Source: CAD feature listing. Evaluate the final solid. Frame: model axes, mm. Give positions to 0.01 mm unless a question says otherwise; leave off trailing zeros. Order: outer loops, then holes, each group sorted by start corner. A loop starts at its lowest first (then second) coordinate and runs counter-clockwise, first axis right, second up. Notation, with made-up numbers: (40, 49) -> (95, 49) arc R16 cw to (95, 76) -> close; hole circle Ø10 at (-37.75, -40). An arc over 180 degrees is marked (long way). Use CSV: the item, a comma, the result in double quotes.
```python
from build123d import *

# Parameters (mm, degrees)
F0_W     = 381
F0_H     = 381
F1_DEPTH = 2.54
F2_R     = 19.05
F3_DEPTH = 2.541


with BuildPart() as f1:
    # F0 (on Front) → F1 (new body)
    with BuildSketch(Plane.XZ):
        with Locations((1.796125, 1.474147)):
            Rectangle(F0_W, F0_H)
    extrude(amount=F1_DEPTH)

    # F2 (on face) → F3 (cut, through all)
    with BuildSketch(Plane.XZ.offset(2.54)):
        Circle(F2_R)
        with Locations((-84.602214, -27.307058)):
            Circle(F2_R)
    extrude(amount=-F3_DEPTH, mode=Mode.SUBTRACT)


solid = f1.part
```
1. Pin query (flat end, axial travel): P1, Ø8, axis at x = -91.5, z = 92.5, coming from the +Y side. Return the tip coordinate at first contact, or that it passes through.
Answer below:
P1,"stops at y = 0"
2. Section query B-B on x = 0. Return loops of the section in (y, z), plus the area to 3 significant figures.
Answer below:
outline,"(-2.54, -189.03) -> (0, -189.03) -> (0, -19.05) -> (-2.54, -19.05) -> close; (-2.54, 19.05) -> (0, 19.05) -> (0, 191.97) -> (-2.54, 191.97) -> close"
area,"871 mm²"
3. Section query A-A on z = 0. Return loops of the section in (x, y).
Answer below:
outline,"(-188.7, -2.54) -> (-19.05, -2.54) -> (-19.05, 0) -> (-188.7, 0) -> close; (19.05, -2.54) -> (192.3, -2.54) -> (192.3, 0) -> (19.05, 0) -> close"
4. Ray query, line 1 along Z through (x, y) = (0, -1.15); line 2 along X through (y, z) = (-0.2, 5.5); line 3 along Z through (x, y) = (-81.5, -2.05). Return the intervals inside material, ascending.
Answer below:
line 1,"z = -189.03 to -19.05, 19.05 to 191.97"
line 2,"x = -188.7 to -18.24, 18.24 to 192.3"
line 3,"z = -189.03 to -46.1, -8.51 to 191.97"
5. Mould query, pull axis Z, two halves, no side actions, for faces 1 (the flat face through (41, 0, 4)), 2 (the cylindrical face through (-103.634, -1.288, -26.469)). Classes: released by +Z, released by -Z, zero draft, split by the parting line, or undercut.
Answer below:
face 1,"zero draft"
face 2,"undercut"
6. Section query C-C on y = -1.65. Return loops of the section in (x, z).
Answer below:
outline,"(-188.7, -189.03) -> (192.3, -189.03) -> (192.3, 191.97) -> (-188.7, 191.97) -> close; hole circle Ø38.1 at (-84.6, -27.31); hole circle Ø38.1 at (0, 0)"
